Input: part model. Units: mm. Frame: model coordinates. Face numbers are marked on the shaded views. A direction names the side the tool comes from. Round coordinates to 2 decimals unless told otherwise and drop trailing zeros. Loops run counter-clockwise (first coordinate to the right, second up) from the corner with the lowest first, then second, coordinate; pieces in that order, holes last. Notation, with made-up numbers: (-27.5, -22) -> (21.5, -22) arc R7 cw to (21.5, -14) -> close; hole circle Ø10 at (-32.5, 57.25). An arc over 180 degrees is marked (long way). Answer as a JSON object with one key per item and string values.
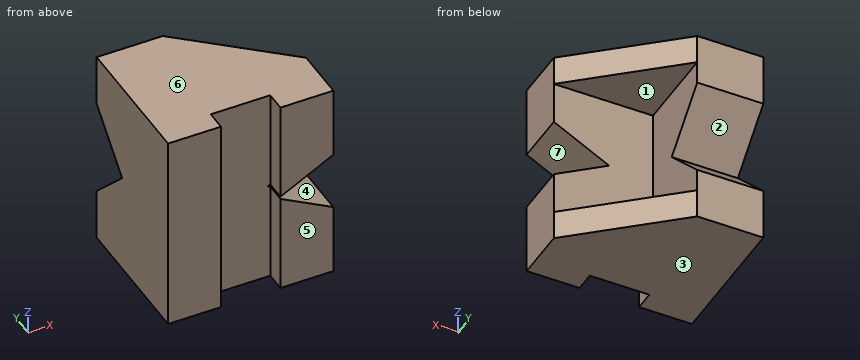
```python
from build123d import *

# Parameters (mm, degrees)
BOSS_EXTRUDE1_DEPTH = 31
BOSS_EXTRUDE3_START = 22
BOSS_EXTRUDE3_DEPTH = 9
BOSS_EXTRUDE4_START = -22
BOSS_EXTRUDE4_DEPTH = 9
CUT_EXTRUDE1_REACH  = 62.208
CUT_EXTRUDE2_REACH  = 66.32


with BuildPart() as part:
    # Sketch1 → Boss-Extrude1 (new, symmetric)
    with BuildSketch(Plane.XY):
        Polygon((16, 0), (0, 0), (0, 42), (20, 42), (20, 16), (50, 16), (50, 0), (34, 0), (34, 6), (16, 6), align=None)
    extrude(amount=BOSS_EXTRUDE1_DEPTH, both=True)

    # Sketch1_7 → Boss-Extrude3 (add)
    with BuildSketch(Plane.XY.offset(BOSS_EXTRUDE3_START)):
        Polygon((20, 16), (50, 16), (20, 42), align=None)
    extrude(amount=BOSS_EXTRUDE3_DEPTH)

    # Sketch1_8 → Boss-Extrude4 (add)
    with BuildSketch(Plane.XY.offset(BOSS_EXTRUDE4_START)):
        Polygon((20, 16), (50, 16), (20, 42), align=None)
    extrude(amount=-BOSS_EXTRUDE4_DEPTH)

    # Sketch2 → Cut-Extrude1 (cut, up to next)
    with BuildSketch(Plane(origin=(20, 0, 0), x_dir=(0, 0, -1), z_dir=(1, 0, 0)), mode=Mode.PRIVATE) as cut_extrude1_sk1:
        Polygon((-15, 42), (0, 27), (15, 42), align=None)
    cut_extrude1_tool1 = extrude(cut_extrude1_sk1.sketch, amount=-CUT_EXTRUDE1_REACH, mode=Mode.PRIVATE) & part.part
    add(cut_extrude1_tool1.solids().sort_by_distance((20, 37, 0))[0], mode=Mode.SUBTRACT)

    # Sketch3 → Cut-Extrude2 (cut, up to next)
    with BuildSketch(Plane(origin=(0, 16, 0), x_dir=(1, 0, 0), z_dir=(0, 1, 0)), mode=Mode.PRIVATE) as cut_extrude2_sk1:
        Polygon((50, 9), (33.300468379, 0), (50, -9), align=None)
    cut_extrude2_tool1 = extrude(cut_extrude2_sk1.sketch, amount=-CUT_EXTRUDE2_REACH, mode=Mode.PRIVATE) & part.part
    add(cut_extrude2_tool1.solids().sort_by_distance((44.433489, 16, 0))[0], mode=Mode.SUBTRACT)


solid = part.part
```
1) Section A-A, the plane y = 29. Output: boundary loops of the cut face in (x, z), plus the area to 3 significant figures.
Output:
{"outline": "(0, -31) -> (35, -31) -> (35, -22) -> (20, -22) -> (20, -2) -> (0, -2) -> close; (0, 2) -> (20, 2) -> (20, 22) -> (35, 22) -> (35, 31) -> (0, 31) -> close", "area": "1,430 mm^2"}
2) Section D-D, the plane x = 38. Output: boundary loops of the cut face in (y, z).
Output:
{"outline": "(0, -31) -> (26.4, -31) -> (26.4, -22) -> (16, -22) -> (16, -2.53) -> (0, -2.53) -> close; (0, 2.53) -> (16, 2.53) -> (16, 22) -> (26.4, 22) -> (26.4, 31) -> (0, 31) -> close"}
3) Ray query, probe 1 along Z at (x, y) = (30, 29.5); probe 2 along X at (y, z) = (4, -14); probe 3 along Y at (x, z) = (28, -4). Return the intervals inside material, ascending.
Output:
{"probe 1": "z = -31 to -22, 22 to 31", "probe 2": "x = 0 to 16, 34 to 50", "probe 3": "y = 6 to 16"}
4) Section B-B, the plane z = 23. Output: boundary loops of the cut face in (x, y), plus the area to 3 significant figures.
Output:
{"outline": "(0, 0) -> (16, 0) -> (16, 6) -> (34, 6) -> (34, 0) -> (50, 0) -> (50, 16) -> (20, 42) -> (0, 42) -> close", "area": "1,600 mm^2"}
5) Reachability of the marked faces 1, 2 and 3 from +Z, -Z, +X, -X, +Y, -Y: full face, straight path, thin tool, end or side. Return the list, or none.
Output:
{"face 1": "+X, +Y", "face 2": "+X, -X, +Y", "face 3": "-Z, +X, -X, +Y, -Y"}
6) Contact query for flat-ended pins moving along their axis: P1, Ø8, axis at x = 5.5, z = 4, coming from the +Y side; P2, Ø14.5, axis at x = 24, z = -4.5, coming from the -Y side; P3, Ø12, axis at y = 31.5, z = 20.5, coming from the +X side. Output: stop coordinate, or through.
Output:
{"P1": "stops at y = 35", "P2": "stops at y = 6", "P3": "stops at x = 38.82"}
7) Draft query along Z for the marked faces 4, 5, 6 and 7. Return one class per face: +Z half, -Z half, draft (parallel to the pull), parting line (faces both ways), or undercut.
Output:
{"face 4": "undercut", "face 5": "draft", "face 6": "+Z half", "face 7": "undercut"}
8) Section C-C, the plane x = 5. Output: boundary loops of the cut face in (y, z), plus the area to 3 significant figures.
Output:
{"outline": "(0, -31) -> (42, -31) -> (42, -15) -> (27, 0) -> (42, 15) -> (42, 31) -> (0, 31) -> close", "area": "2,380 mm^2"}
